Geometry: final body of the model. Coordinates: model frame, mm. A direction names the side the tool comes from. Round coordinates to 2 decimals unless told otherwise and drop trailing zeros. Put each result on its own line as item: value. Start each with the question number.
1) First-contact query: P1, Ø4, axis at y = 12.7, z = 1574.8, coming from the -X side (3 decimals); P2, Ø3, axis at y = 12.7, z = 1581.15, coming from the +X side (3 decimals); P3, Ø3, axis at y = 12.7, z = 1562.1, coming from the -X side. Flat tips, straight axial feed; report the tip coordinate or a pass-through.
2) Draft query along X for faces 1 (the flat face through (12.5, 23.8, 1815.9)), 2 (the cylindrical face through (13.425, 23.79, 1747.758)), 3 (the cylindrical face through (1.57, 13.42, 1538.97)). Return one class per face: pulls with the +X half, pulls with the -X half, needs draft (parallel to the pull), parting line crosses it, or undercut.
3) Material intervals for probe 1 along X at (y, z) = (13.75, 1780.5) (3 decimals); probe 2 along Y at (x, z) = (0.7, 1536.7), sorted ascending. Write a range as [from, to].
4) Access query for faces 4 (the cylindrical face through (1.57, 13.42, 1589.77)), 5 (the cylindrical face through (11.232, 1.61, 1805.656)), 6 (the flat face through (3.175, 13, 1663)). Directions: +Z, -Z, +X, -X, +Y, -Y. A direction counts if a zero-diameter tool reaches every point of the face in a straight line with its end or side. Return the directions, or none.
from build123d import *

# Parameters (mm, degrees)
CUT_EXTRUDE1_START = 1524
CUT_EXTRUDE1_DEPTH = 304.8
CUT_EXTRUDE2_START = -25.4
CUT_EXTRUDE2_DEPTH = 25.4
SKETCH3_R          = 2.413
CUT_EXTRUDE3_DEPTH = 1830.152743759
SKETCH4_R          = 2.413
CUT_EXTRUDE4_DEPTH = 1830.152743759
CUT_EXTRUDE5_REACH = 1831.153
SKETCH5_R          = 2.38125
CUT_EXTRUDE6_REACH = 1831.153
SKETCH6_R          = 2.38125


with BuildPart() as part:
    # Cut-Extrude1: read off the stored shape, not the designer's step
    # Cut-Extrude1 outline → Cut-Extrude1 (new body)
    with BuildSketch(Plane.XY.offset(CUT_EXTRUDE1_START)):
        with BuildLine():
            Line((0, 25.146), (0, 0.254))
            ThreePointArc((0, 0.254), (0.074394878, 0.074394878), (0.254, 0))
            Line((0.254, 0), (25.146, 0))
            ThreePointArc((25.146, 0), (25.325605122, 0.074394878), (25.4, 0.254))
            Line((25.4, 0.254), (25.4, 25.146))
            ThreePointArc((25.4, 25.146), (25.325605122, 25.325605122), (25.146, 25.4))
            Line((25.146, 25.4), (0.254, 25.4))
            ThreePointArc((0.254, 25.4), (0.074394878, 25.325605122), (0, 25.146))
        make_face()
        with BuildLine():
            ThreePointArc((4.7625, 3.175), (3.639967985, 3.639967985), (3.175, 4.7625))
            Line((3.175, 4.7625), (3.175, 20.6375))
            ThreePointArc((3.175, 20.6375), (3.639967985, 21.760032015), (4.7625, 22.225))
            Line((4.7625, 22.225), (20.6375, 22.225))
            ThreePointArc((20.6375, 22.225), (21.760032015, 21.760032015), (22.225, 20.6375))
            Line((22.225, 20.6375), (22.225, 4.7625))
            ThreePointArc((22.225, 4.7625), (21.760032015, 3.639967985), (20.6375, 3.175))
            Line((20.6375, 3.175), (4.7625, 3.175))
        make_face(mode=Mode.SUBTRACT)
    extrude(amount=CUT_EXTRUDE1_DEPTH)

    # Sketch2 → Cut-Extrude2 (cut)
    with BuildSketch(Plane(origin=(0, 25.4, 0), x_dir=(1, 0, 0), z_dir=(0, 1, 0)).offset(CUT_EXTRUDE2_START)):
        Polygon((-15.751867444, -1787.648132556), (56.090181524, -1859.490181524), (20.16915704, -1895.411206008), (-51.672891929, -1823.56915704), align=None)
    extrude(amount=CUT_EXTRUDE2_DEPTH, mode=Mode.SUBTRACT)

    # Sketch3 → Cut-Extrude3 (cut, through all)
    with BuildSketch(Plane.XZ):
        with Locations(Location((12.7, 1536.7, 0), (0, 0, 270))):
            Circle(SKETCH3_R)
        with Locations(Location((12.7, 1607.82, 0), (0, 0, 270))):
            Circle(SKETCH3_R)
        with Locations(Location((12.7, 1678.94, 0), (0, 0, 270))):
            Circle(SKETCH3_R)
        with Locations(Location((12.7, 1750.06, 0), (0, 0, 270))):
            Circle(SKETCH3_R)
    extrude(amount=-CUT_EXTRUDE3_DEPTH, mode=Mode.SUBTRACT)

    # Sketch4 → Cut-Extrude4 (cut, through all)
    with BuildSketch(Plane(origin=(0, 25.4, 0), x_dir=(1, 0, 0), z_dir=(0, 1, 0))):
        with Locations(Location((12.7, -1807.571024484, 0), (0, 0, 270))):
            Circle(SKETCH4_R)
        with Locations(Location((12.7, -1788.521024484, 0), (0, 0, 270))):
            Circle(SKETCH4_R)
    extrude(amount=-CUT_EXTRUDE4_DEPTH, mode=Mode.SUBTRACT)

    # Sketch5 → Cut-Extrude5 (cut, up to next)
    with BuildSketch(Plane.ZY, mode=Mode.PRIVATE) as cut_extrude5_sk1:
        with Locations((1536.7, 12.7)):
            Circle(SKETCH5_R)
    cut_extrude5_tool1 = extrude(cut_extrude5_sk1.sketch, amount=-CUT_EXTRUDE5_REACH, mode=Mode.PRIVATE) & part.part
    # Sketch5 → Cut-Extrude5 (cut, up to next)
    with BuildSketch(Plane.ZY, mode=Mode.PRIVATE) as cut_extrude5_sk2:
        with Locations((1549.4, 12.7)):
            Circle(SKETCH5_R)
    cut_extrude5_tool2 = extrude(cut_extrude5_sk2.sketch, amount=-CUT_EXTRUDE5_REACH, mode=Mode.PRIVATE) & part.part
    # Sketch5 → Cut-Extrude5 (cut, up to next)
    with BuildSketch(Plane.ZY, mode=Mode.PRIVATE) as cut_extrude5_sk3:
        with Locations((1562.1, 12.7)):
            Circle(SKETCH5_R)
    cut_extrude5_tool3 = extrude(cut_extrude5_sk3.sketch, amount=-CUT_EXTRUDE5_REACH, mode=Mode.PRIVATE) & part.part
    # Sketch5 → Cut-Extrude5 (cut, up to next)
    with BuildSketch(Plane.ZY, mode=Mode.PRIVATE) as cut_extrude5_sk4:
        with Locations((1574.8, 12.7)):
            Circle(SKETCH5_R)
    cut_extrude5_tool4 = extrude(cut_extrude5_sk4.sketch, amount=-CUT_EXTRUDE5_REACH, mode=Mode.PRIVATE) & part.part
    # Sketch5 → Cut-Extrude5 (cut, up to next)
    with BuildSketch(Plane.ZY, mode=Mode.PRIVATE) as cut_extrude5_sk5:
        with Locations((1587.5, 12.7)):
            Circle(SKETCH5_R)
    cut_extrude5_tool5 = extrude(cut_extrude5_sk5.sketch, amount=-CUT_EXTRUDE5_REACH, mode=Mode.PRIVATE) & part.part
    add(cut_extrude5_tool1.solids().sort_by_distance((0, 12.7, 1536.7))[0], mode=Mode.SUBTRACT)
    add(cut_extrude5_tool2.solids().sort_by_distance((0, 12.7, 1549.4))[0], mode=Mode.SUBTRACT)
    add(cut_extrude5_tool3.solids().sort_by_distance((0, 12.7, 1562.1))[0], mode=Mode.SUBTRACT)
    add(cut_extrude5_tool4.solids().sort_by_distance((0, 12.7, 1574.8))[0], mode=Mode.SUBTRACT)
    add(cut_extrude5_tool5.solids().sort_by_distance((0, 12.7, 1587.5))[0], mode=Mode.SUBTRACT)

    # Sketch6 → Cut-Extrude6 (cut, up to next)
    with BuildSketch(Plane(origin=(25.4, 0, 0), x_dir=(0, 0, -1), z_dir=(1, 0, 0)), mode=Mode.PRIVATE) as cut_extrude6_sk1:
        with Locations(Location((-1562.1, 12.7, 0), (0, 0, 180))):
            Circle(SKETCH6_R)
    cut_extrude6_tool1 = extrude(cut_extrude6_sk1.sketch, amount=-CUT_EXTRUDE6_REACH, mode=Mode.PRIVATE) & part.part
    # Sketch6 → Cut-Extrude6 (cut, up to next)
    with BuildSketch(Plane(origin=(25.4, 0, 0), x_dir=(0, 0, -1), z_dir=(1, 0, 0)), mode=Mode.PRIVATE) as cut_extrude6_sk2:
        with Locations((-1581.15, 12.7)):
            Circle(SKETCH6_R)
    cut_extrude6_tool2 = extrude(cut_extrude6_sk2.sketch, amount=-CUT_EXTRUDE6_REACH, mode=Mode.PRIVATE) & part.part
    add(cut_extrude6_tool1.solids().sort_by_distance((25.4, 12.7, 1562.1))[0], mode=Mode.SUBTRACT)
    add(cut_extrude6_tool2.solids().sort_by_distance((25.4, 12.7, 1581.15))[0], mode=Mode.SUBTRACT)


solid = part.part
Result sheet:
1. P1: stops at x = 22.225
1. P2: stops at x = 3.175
1. P3: passes through
2. face 1: pulls with the -X half
2. face 2: undercut
2. face 3: needs draft
3. probe 1: x = [0, 3.175], [22.225, 25.4]
3. probe 2: y = [0, 10.32], [15.08, 25.4]
4. face 4: -X
4. face 5: +Y, -Y
4. face 6: +Z, -Z
